Design review of the part shown in the three views and the two pictorial views. Dimensions are in mm from the part's minimum x, y and z. Give positions to 0.01 mm unless a question says otherwise; leave off trailing zeros. Order: outer loops, then holes, each group sorted by start corner. A loop starts at its lowest first (then second) coordinate and runs counter-clockwise, first axis right, second up. Notation, with made-up numbers: M 11,85 L 23,85 A11 cw 23,93 Z; hole C -17.75,53 d8. An arc over 180 degrees is marked long. Answer as a JSON object with one key per item and string values.
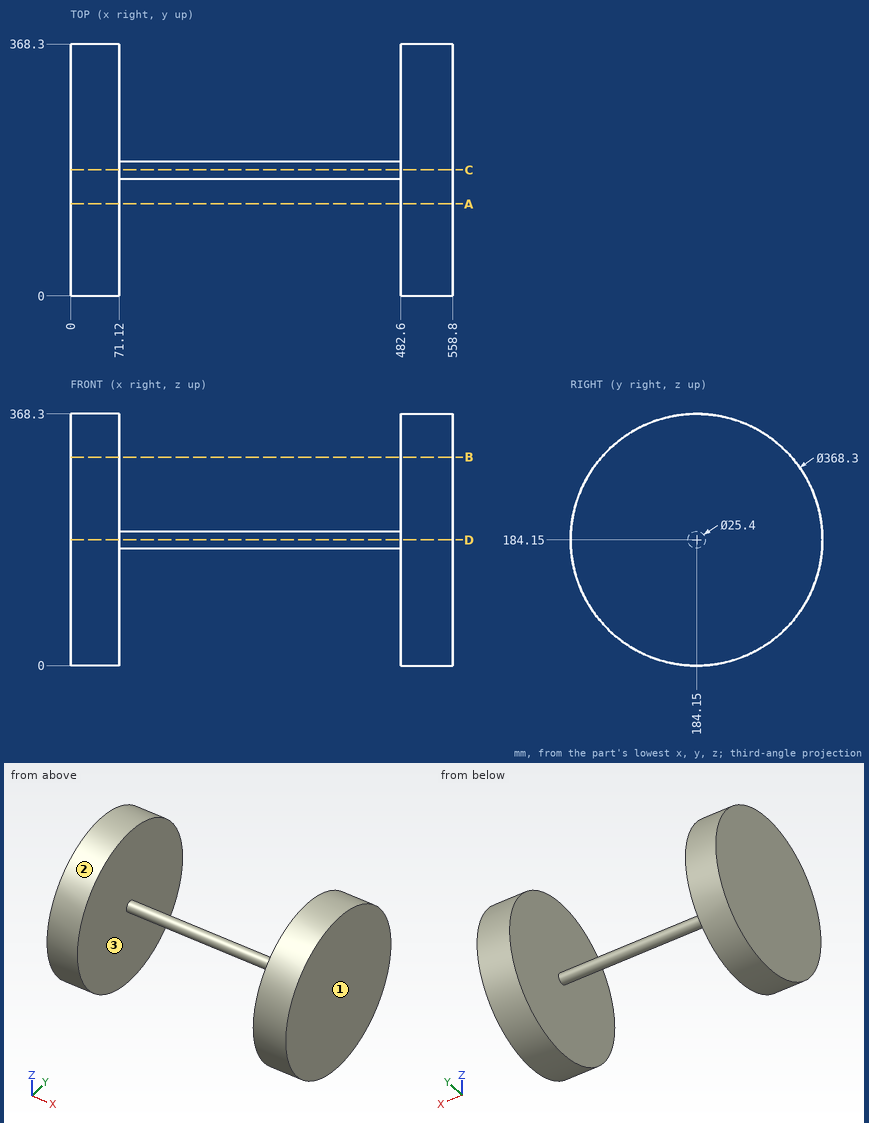
(1) To check wall thickness, follow L1, parallel to X at y = 231, z = 80.5; L2, parallel to Y at x = 31, z = 205; L3, parallel to Y at x = 499, z = 246.5. State the ranges of each line that lie inside material, in increasing order. Write a range as from..to.
Checked values:
{"L1": "x = 0..71.12, 482.6..558.8", "L2": "y = 1.18..367.12", "L3": "y = 10.88..357.42"}
(2) We need section A-A (y = 134.5). Write out the cut boundary in (x, z), plus the area to 3 significant figures.
Checked values:
{"outline": "M 0,6.82 L 71.12,6.82 L 71.12,361.48 L 0,361.48 Z; M 482.6,6.82 L 558.8,6.82 L 558.8,361.48 L 482.6,361.48 Z", "area": "52,200 mm^2"}
(3) Insertion check: pin 1 (12 mm diameter, centred on y = 96, z = 90.5, fed in from -X). The pin has a flat end and moves straight along its axis. Give the tip position at first contact, or say it passes through.
Checked values:
{"pin 1": "stops at x = 0"}
(4) We need section B-B (z = 305). Write out the cut boundary in (x, y).
Checked values:
{"outline": "M 0,45.2 L 71.12,45.2 L 71.12,323.1 L 0,323.1 Z; M 482.6,45.2 L 558.8,45.2 L 558.8,323.1 L 482.6,323.1 Z"}
(5) We need section C-C (y = 184.15). Write out the cut boundary in (x, z).
Checked values:
{"outline": "M 0,0 L 71.12,0 L 71.12,171.45 L 482.6,171.45 L 482.6,0 L 558.8,0 L 558.8,368.3 L 482.6,368.3 L 482.6,196.85 L 71.12,196.85 L 71.12,368.3 L 0,368.3 Z"}
(6) Draft analysis for pull direction X (two halves, no side actions). For the marked faces 1, 2 and 3, state which applies: +X half, -X half, draft (parallel to the pull), parting line (faces both ways), or undercut.
Checked values:
{"face 1": "+X half", "face 2": "draft", "face 3": "undercut"}
